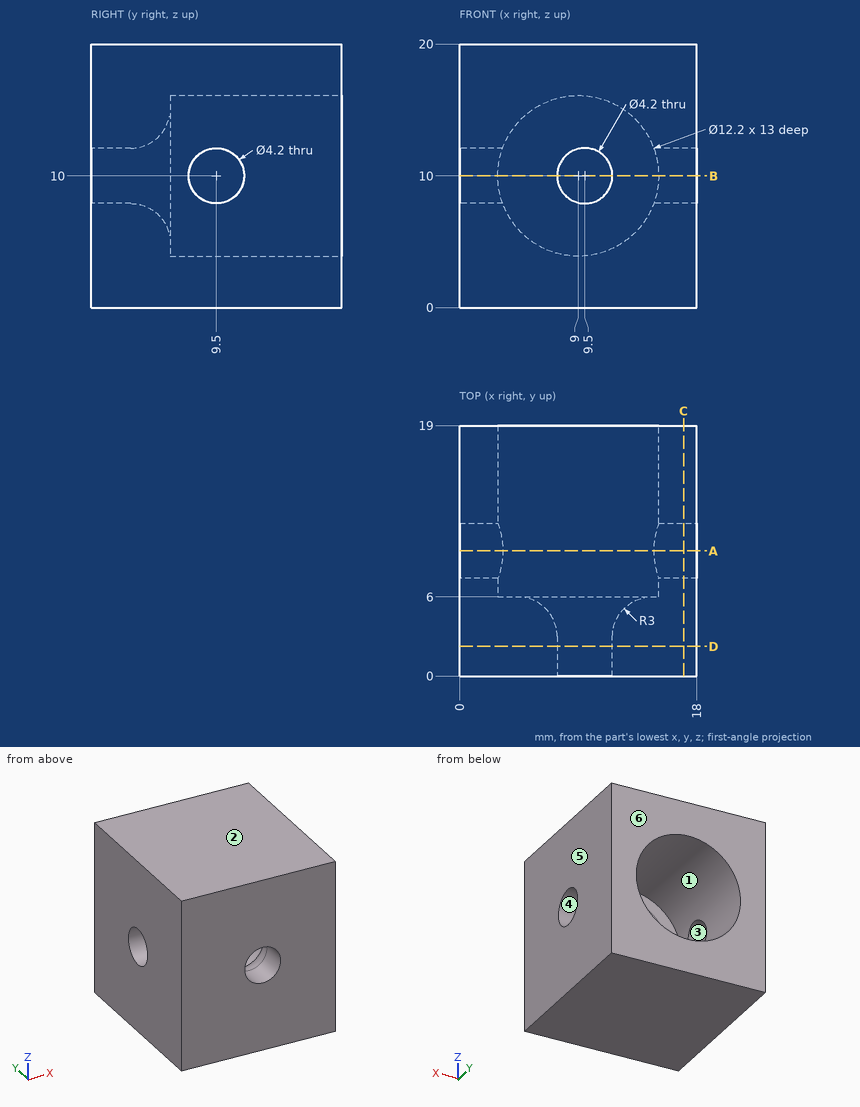
Print and shaded views of the part. All mm, measured from the part's lowest x, y and z. A direction names the side the tool comes from. Round coordinates to 2 decimals unless told otherwise and drop trailing zeros. Write each loop counter-clockwise with the first axis right and the second up, starting at its lowest first coordinate (ties: lowest second). Pieces come first, ordered by that corner, then holes. Notation, with made-up numbers: (58, 71.5) - (96, 71.5) arc R13 cw to (96, 93.5) - close; hole circle Ø5 at (78, 34.25). An arc over 180 degrees is marked (long way). Write each question's results on one line, items separated by ' | '. Start each with the question number.
Item 1: Saw through at B-B (z = 10). Write the cut outline in (x, y).
Item 2: Saw through at C-C (x = 17). Write the cut outline in (y, z), and give its area (3 significant figures).
Item 3: Saw through at D-D (y = 2.25). Write the cut outline in (x, z).
Item 4: Wall check: L1, parallel to Y at x = 2.5, z = 10; L2, parallel to Z at x = 16.4, y = 9.5; L3, parallel to Z at x = 4.75, y = 15.5. Give the ranges that are in metal, low to high. Write a range as [from, to].
Item 5: Which spindle directions (+Z, -Z, +X, -X, +Y, -Y) get a long thin tool onto all of the face, cutting with end or side? Do the marked faces 1 and 2. Say none if no direction does.
Item 6: Mould opens along Y. For the marked faces 3, 4, 5 and 6 say: pulls with the +Y half, pulls with the -Y half, needs draft (parallel to the pull), parting line crosses it, or undercut.
Item 7: Drop flat-ended pins along their axis: P1, Ø3.5, axis at x = 9.5, z = 10, coming from the +Y side; P2, Ø5, axis at x = 12, z = 11.5, coming from the +Y side; P3, Ø7.5, axis at x = 9, z = 10, coming from the +Y side. Give the stop position or say it passes through.
Item 8: Saw through at A-A (y = 9.5). Write the cut outline in (x, z).
Results are:
1) outline: (0, 0) - (7.4, 0) - (7.4, 3) arc R3 ccw to (4.4, 6) - (2.9, 6) - (2.9, 7.4) - (0, 7.4) - close; (0, 11.6) - (2.9, 11.6) - (2.9, 19) - (0, 19) - close; (11.6, 0) - (18, 0) - (18, 7.4) - (15.1, 7.4) - (15.1, 6) - (14.6, 6) arc R3 ccw to (11.6, 3) - close; (15.1, 11.6) - (18, 11.6) - (18, 19) - (15.1, 19) - close
2) outline: (0, 0) - (19, 0) - (19, 20) - (0, 20) - close; hole circle Ø4.2 at (9.5, 10) | area: 366 mm²
3) outline: (0, 0) - (18, 0) - (18, 20) - (0, 20) - close; hole circle Ø4.2 at (9.5, 10)
4) L1: y = [0, 7.4], [11.6, 19] | L2: z = [0, 7.9], [12.1, 20] | L3: z = [0, 5.62], [14.38, 20]
5) face 1: +Y | face 2: +Z, +X, -X, +Y, -Y
6) face 3: undercut | face 4: undercut | face 5: needs draft | face 6: pulls with the +Y half
7) P1: passes through | P2: stops at y = 6 | P3: stops at y = 5.88
8) outline: (0, 0) - (18, 0) - (18, 7.9) - (14.73, 7.9) arc R6.1 cw to (3.27, 7.9) - (0, 7.9) - close; (0, 12.1) - (3.27, 12.1) arc R6.1 cw to (14.73, 12.1) - (18, 12.1) - (18, 20) - (0, 20) - close
